Geometry check sheet. Reference: the model listing, model coordinates, mm. Coordinates: 2 decimals unless noted, no trailing zeros. Order: outer loops, then holes, each group sorted by start corner. A loop starts at its lowest first (then second) coordinate and runs counter-clockwise, first axis right, second up. Notation, with made-up numbers: M 58,22.25 L 75,22.25 A23 ccw 75,53.25 Z; hole C -25,4 d8. An arc over 180 degrees is marked long. One line per item, written item: value. Start each with the question number.
1) Sectioned sample at B-B, the plane z = 214. Enter the section's corners in (x, y), then the cut area to 3 significant figures.
2) Thickness scan on L1, parallel to X at y = 8.25, z = 20; L2, parallel to Z at x = 511, y = 9.5. Record the ranges inside material, lowest first. Write a range as from..to.
3) Go/stop test with a flat-tipped pin: P1, Ø8, axis at x = 419.82, z = 378, coming from the -Y side. Record where the tip stops, or that it passes through.
4) Sectioned sample at A-A, the plane x = 220. Enter the section's corners in (y, z).
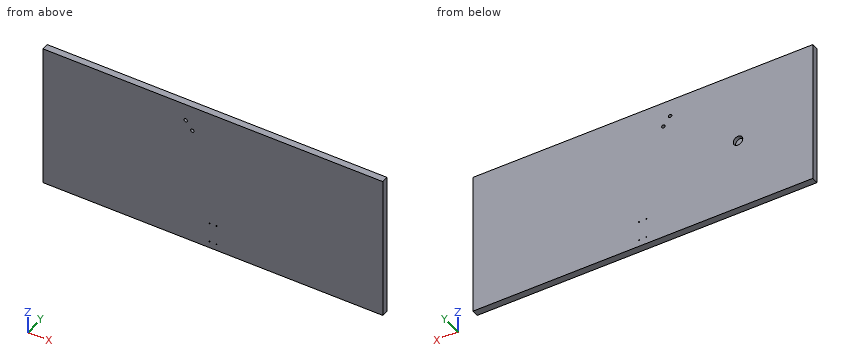
Autodesk Inventor part; units mm, degrees
ref_plane "YZ Plane" through (0, 0, 0) normal (1, 0, 0) x (0, 1, 0)
ref_plane "XZ Plane" through (0, 0, 0) normal (0, 1, 0) x (-1, 0, 0)
ref_plane "XY Plane" through (0, 0, 0) normal (0, 0, 1) x (1, 0, 0)
sketch "Skizze1" plane through (0, 0, 0) normal (0, 1, 0) x (-1, 0, 0)
  line L0 (0, 0) -> (-1000, 0)
  line L1 (-1000, 0) -> (-1000, 428)
  line L2 (-1000, 428) -> (0, 428)
  line L3 (0, 428) -> (0, 0)
  dimension "d0" = 1000
  dimension "d1" = 428
extrude "Extrusion1" add sketch "Skizze1" along normal blind 20
sketch "Skizze2" plane through (0, 20, 0) normal (0, 1, 0) x (1, 0, 0)
  line L0 (0, 0) -> (0, -428)
  line L1 (0, -428) -> (220, -428)
  line L2 (220, -428) -> (220, -214)
  circle A0 centre (220, -214) radius 14
  dimension "d4" = 220
  dimension "d5" = 214
  dimension "d6" = 28
extrude "Extrusion2" cut sketch "Skizze2" against normal blind 11
sketch "Skizze3" plane through (0, 20, 0) normal (0, 1, 0) x (1, 0, 0)
  line L0 (0, -429.5296) -> (419.9972, -428)
  line L1 (0, -428) -> (1000, -428)
  line L2 (419.9972, -428) -> (419.8151, -378.0003)
  line L3 (419.8151, -378.0003) -> (439.815, -377.9275)
  line L4 (439.815, -377.9275) -> (439.7239, -352.9277)
  point P0 (0, 0)
  dimension "d9" = 420
  dimension "d10" = 50
  dimension "d11" = 20
  dimension "d12" = 25
hole "Bohrung1" at (419.8151, 20, 378.0003) at (439.7239, 20, 352.9277) direction (0, -1, 0) diameter 10 depth 20 tip angle 118
sketch "Skizze4" plane through (0, 20, 0) normal (0, 1, 0) x (1, 0, 0)
  line L0 (1000, 0) -> (0, 0)
  line L1 (0, 0) -> (490, 0)
  line L2 (490, 0) -> (505, 0)
  line L3 (490, 0) -> (490, -15)
  line L4 (490, -15) -> (490, -20)
  circle A0 centre (490, -20) radius 1.5
  line L5 (490, -20) -> (511, -20)
  circle A1 centre (511, -20) radius 1.5
  dimension "d20" = 490
  dimension "d22" = 15
  dimension "d23" = 5
  dimension "d24" = 3
  dimension "d25" = 21
  dimension "d26" = 3
hole "Bohrung2" at (490, 20, 20) at (511, 20, 20) direction (0, -1, 0) diameter 3 end through all
sketch "Skizze5" plane through (0, 20, 0) normal (0, 1, 0) x (1, 0, 0)
  circle A0 centre (490, -20) radius 1.5
  line L0 (490, -20) -> (490, -78)
  circle A1 centre (511, -20) radius 1.5
  line L1 (511, -20) -> (511, -78)
  point P0 (0, 0)
  dimension "d34" = 58
  dimension "d35" = 58
hole "Bohrung3" at (511, 20, 78) at (490, 20, 78) direction (0, -1, 0) diameter 3 end through all
properties part number "Grundplatte" material "Holz (Birke)"
Final values:
1. outline: M 0,0 L 1000,0 L 1000,20 L 234,20 L 234,9 L 206,9 L 206,20 L 0,20 Z
1. area: 19,700 mm^2
2. L1: x = 0..488.5, 491.5..509.5, 512.5..1000
2. L2: z = 0..18.5, 21.5..76.5, 79.5..428
3. P1: passes through
4. outline: M 0,0 L 20,0 L 20,200 L 9,200 L 9,228 L 20,228 L 20,428 L 0,428 Z
